Work out the finished part from the listing and answer in its coordinate system (mm). Face numbers are marked on the shaded views. A direction names the side the tool comes from. Coordinates: 2 decimals unless noted, no trailing zeros. Write each loop counter-clockwise with the first axis right and the second up, starting at its lowest first coordinate (ties: lowest second). Pieces come first, ordered by that corner, then holes. Notation, with made-up numbers: M 62,80.5 L 104,80.5 A3 ccw 104,84.5 Z; hole C -25,26 d10. An arc over 180 degrees is marked long. Use CSV: the item, a comma, the result in double quotes.
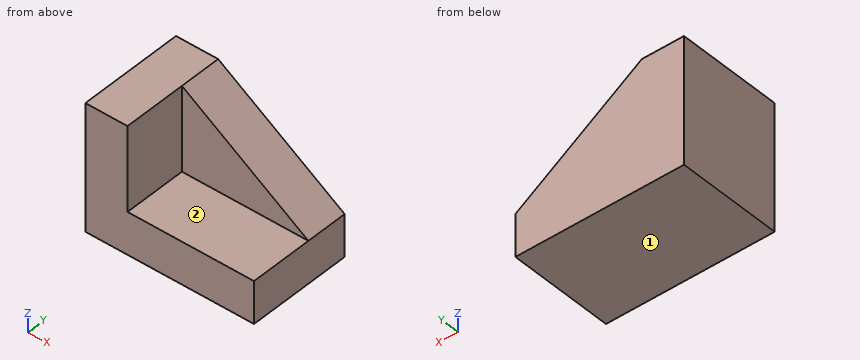
from build123d import *

# Parameters (mm, degrees)
F1_DEPTH = 63.5
F3_DEPTH = 38.1


with BuildPart() as f1:
    # F0 (on Front) → F1 (new body)
    with BuildSketch(Plane.XZ):
        Polygon((57.172726, -32.42728), (-19.027274, 18.37272), (-44.427274, 18.37272), (-44.427274, -57.82728), (57.172726, -57.82728), align=None)
    extrude(amount=F1_DEPTH)

    # F2 (on face) → F3 (cut)
    with BuildSketch(Plane.XZ.offset(63.5)):
        Polygon((-19.027274, 18.37272), (-19.027274, -32.42728), (57.172726, -32.42728), align=None)
    extrude(amount=-F3_DEPTH, mode=Mode.SUBTRACT)


solid = f1.part
Item 1: The part is cut by section B-B (x = 27.5). Write down the section's boundary in (y, z).
Answer:
outline,"M -63.5,-57.83 L 0,-57.83 L 0,-12.65 L -25.4,-12.65 L -25.4,-32.43 L -63.5,-32.43 Z"
Item 2: The part is cut by section A-A (y = -14). Write down the section's boundary in (x, z).
Answer:
outline,"M -44.43,-57.83 L 57.17,-57.83 L 57.17,-32.43 L -19.03,18.37 L -44.43,18.37 Z"
Item 3: The part is cut by section C-C (z = -6.5). Write down the section's boundary in (x, y), then the cut area to 3 significant figures.
Answer:
outline,"M -44.43,-63.5 L -19.03,-63.5 L -19.03,-25.4 L 18.28,-25.4 L 18.28,0 L -44.43,0 Z"
area,"2,560 mm2"
Item 4: A tool of negligible diameter and unlimited length cuts with its end or side. For the marked faces 1 and 2, from which of +Z, -Z, +X, -X, +Y, -Y can it reach the whole face along a straight path? Write none if from no direction.
Answer:
face 1,"-Z, +X, -X, +Y, -Y"
face 2,"+Z, +X, -Y"
Item 5: Consider probe 1 along Z at (x, y) = (51, -44); probe 2 along Y at (x, z) = (-13, 3); probe 3 along X at (y, z) = (-53, -1). Determine where each line is inside the solid, lowest interval first.
Answer:
probe 1,"z = -57.83 to -32.43"
probe 2,"y = -25.4 to 0"
probe 3,"x = -44.43 to -19.03"
Item 6: Given pin 1 (1 mm diameter, centred on y = -18, z = -23.5, fed in from +X); pin 2 (3 mm diameter, centred on y = -57, z = -6.5, fed in from +X); pin 3 (10 mm diameter, centred on x = -12.5, z = 4, fed in from -Y), each flat-ended and moving along its own axis, determine where each tip first touches the part or whether it passes through.
Answer:
pin 1,"stops at x = 44.53"
pin 2,"stops at x = -19.03"
pin 3,"stops at y = -25.4"
